Autodesk Inventor part; units mm, degrees
ref_plane "YZ Plane" through (0, 0, 0) normal (1, 0, 0) x (0, 1, 0)
ref_plane "XZ Plane" through (0, 0, 0) normal (0, 1, 0) x (-1, 0, 0)
ref_plane "XY Plane" through (0, 0, 0) normal (0, 0, 1) x (1, 0, 0)
sketch "Boceto1" plane through (0, 0, 0) normal (1, 0, 0) x (0, 1, 0)
  line L0 (-6.321, 6.321) -> (6.321, 6.321) construction
  line L1 (6.321, 6.321) -> (6.321, -6.321) construction
  line L2 (6.321, -6.321) -> (-6.321, -6.321) construction
  line L3 (-6.321, -6.321) -> (-6.321, 6.321) construction
  line L4 (-6.321, 6.321) -> (6.321, -6.321) construction
  line L5 (6.321, 6.321) -> (-6.321, -6.321) construction
  circle A0 centre (6.321, -6.321) radius 0.875
  line L6 (0, 0) -> (7.9878, 0) construction
  circle A1 centre (6.321, 6.321) radius 0.875
  line L7 (0, 0) -> (0, -13.4562) construction
  circle A2 centre (-6.321, -6.321) radius 0.875
  circle A3 centre (-6.321, 6.321) radius 0.875
  circle A4 centre (0, 0) radius 5.5
  line L8 (10, 20) -> (-20, 20)
  line L9 (-20, 20) -> (-20, -20)
  line L10 (-20, -20) -> (10, -20)
  line L11 (10, -20) -> (10, 20)
  dimension "d0" = 12.642
  dimension "d1" = 12.642
  dimension "d2" = 1.75
  dimension "d3" = 11
  dimension "d4" = 30
  dimension "d6" = 20
  dimension "d7" = 10
  dimension "d26" = 20
extrude "Extrusión1" add sketch "Boceto1" along normal blind 2
sketch "Boceto2" plane through (0, -20, -20) normal (0, -1, 0) x (1, 0, 0)
  line L0 (2, 0) -> (2, 40)
  line L1 (2, 40) -> (-38, 40)
  line L2 (-38, 40) -> (-38, 0)
  line L3 (-38, 0) -> (2, 0)
  line L4 (2, 0) -> (2, 40)
  point P0 (0, 20)
  point P1 (2, 0)
  dimension "d10" = 40
  dimension "d11" = 40
extrude "Extrusión2" add sketch "Boceto2" along normal blind 2
fillet "Empalme1" radius 1.5 1 edges at (0, -20, 0)
fillet "Empalme2" radius 1 5 edges at (1, 10, 20) (1, 10, -20) (-38, -21, 20) (-38, -21, -20) (2, -22, 0)
sketch "Boceto4" plane through (0, -20, -20) normal (0, 1, 0) x (1, 0, 0)
  circle A0 centre (-13, -10) radius 2.5
  circle A1 centre (-13, -30) radius 2.5
  circle A2 centre (-28, -10) radius 2.5
  circle A3 centre (-28, -30) radius 2.5
  line L0 (-1.5, -40) -> (-37, -40)
  line L1 (-38, -39) -> (-38, -1)
  point P0 (0, -20)
  dimension "d27" = 5
  dimension "d28" = 5
  dimension "d29" = 5
  dimension "d30" = 5
  dimension "d31" = 10
  dimension "d32" = 20
  dimension "d33" = 20
  dimension "d34" = 15
  dimension "d35" = 10
extrude "Extrusión4" cut sketch "Boceto4" against normal through all
sketch "Boceto3" plane through (0, -20, -20) normal (0, 1, 0) x (1, 0, 0)
  line L0 (0, -40) -> (0, 0)
  line L1 (-28, 0) -> (0, 0)
  line L2 (-28, -40) -> (-28, 0)
  line L3 (0, -40) -> (-28, -40)
  line L4 (-6.125, -3.125) -> (-6.125, -36.875) construction
  line L5 (-7.25, -3.125) -> (-7.25, -36.875)
  line L6 (-5, -36.875) -> (-5, -3.125)
  arc A0 (-5, -3.125) -> (-7.25, -3.125) centre (-6.125, -3.125) ccw
  arc A1 (-7.25, -36.875) -> (-5, -36.875) centre (-6.125, -36.875) ccw
  line L7 (-21.875, -3.125) -> (-21.875, -36.875) construction
  line L8 (-23, -3.125) -> (-23, -36.875)
  line L9 (-20.75, -36.875) -> (-20.75, -3.125)
  arc A2 (-20.75, -3.125) -> (-23, -3.125) centre (-21.875, -3.125) ccw
  arc A3 (-23, -36.875) -> (-20.75, -36.875) centre (-21.875, -36.875) ccw
  point P0 (0, -20)
  point P1 (-6.125, -20)
  point P2 (-21.875, -20)
  point P3 (-21.875, -38)
  point P4 (-21.875, -2)
  point P5 (-6.125, -38)
  point P6 (-6.125, -2)
  dimension "d14" = 2.25
  dimension "d15" = 2.25
  dimension "d16" = 5
  dimension "d17" = 2
  dimension "d18" = 2
  dimension "d19" = 2
  dimension "d20" = 2
  dimension "d21" = 5
properties part number "BRACKET_MOTOR" material "Aluminio 6061"
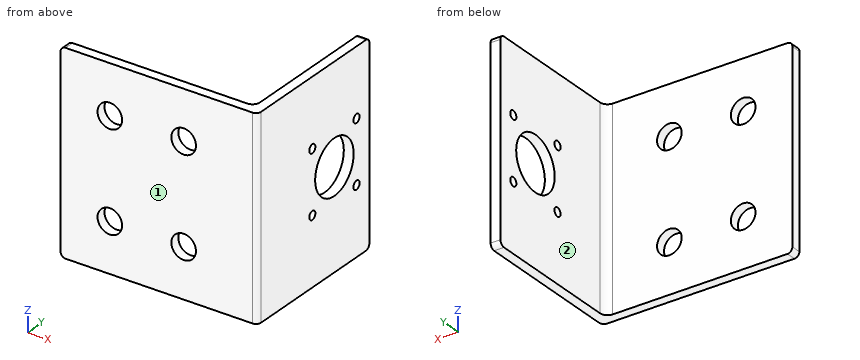
Geometry check sheet. Reference: the model listing, model coordinates, mm. Face numbers are marked on the shaded views. A direction names the side the tool comes from. Give positions to 0.01 mm unless a question says otherwise; leave off trailing zeros. Write each loop counter-clockwise with the first axis right and the second up, starting at its lowest first coordinate (ties: lowest second). Pieces come first, ordered by that corner, then holes. Notation, with made-up numbers: (-27.5, 57) - (-20.5, 57) arc R19 ccw to (-20.5, 62) - close; hole circle Ø11 at (42.25, 47.25). An arc over 180 degrees is marked (long way). Use a Markdown table: item, result.
Q1. Section check D-D, the plane z = 0. Enter the section's corners in (x, y), then the cut area to 3 significant figures.
Computed:
| item | result |
|---|---|
| outline | (-38, -22) - (1, -22) arc R1 ccw to (2, -21) - (2, -5.5) - (0, -5.5) - (0, -18.5) arc R1.5 cw to (-1.5, -20) - (-38, -20) - close; (0, 5.5) - (2, 5.5) - (2, 10) - (0, 10) - close |
| area | 118 mm² |
Q2. Section check C-C, the plane x = -13. Enter the section's corners in (y, z).
Computed:
| item | result |
|---|---|
| outline | (-22, -20) - (-20, -20) - (-20, -12.5) - (-22, -12.5) - close; (-22, -7.5) - (-20, -7.5) - (-20, 7.5) - (-22, 7.5) - close; (-22, 12.5) - (-20, 12.5) - (-20, 20) - (-22, 20) - close |
Q3. Go/stop test with flat-tipped pins: P1, Ø1, axis at x = -32, z = 6.5, coming from the +Y side; P2, Ø14, axis at y = -2.5, z = 2.5, coming from the -X side. Record where each tip stops, or that it passes through.
Computed:
| item | result |
|---|---|
| P1 | stops at y = -20 |
| P2 | stops at x = 0 |
Q4. Section check B-B, the plane y = 0. Enter the section's corners in (x, z), then the cut area to 3 significant figures.
Computed:
| item | result |
|---|---|
| outline | (0, -20) - (2, -20) - (2, -5.5) - (0, -5.5) - close; (0, 5.5) - (2, 5.5) - (2, 20) - (0, 20) - close |
| area | 58.0 mm² |
Q5. Section check A-A, the plane z = 10. Enter the section's corners in (x, y), then the cut area to 3 significant figures.
Computed:
| item | result |
|---|---|
| outline | (-38, -22) - (-30.5, -22) - (-30.5, -20) - (-38, -20) - close; (-25.5, -22) - (-15.5, -22) - (-15.5, -20) - (-25.5, -20) - close; (-10.5, -22) - (1, -22) arc R1 ccw to (2, -21) - (2, 10) - (0, 10) - (0, -18.5) arc R1.5 cw to (-1.5, -20) - (-10.5, -20) - close |
| area | 120 mm² |
Q6. Set-up check for the marked faces 1 and 2: record each of +Z, -Z, +X, -X, +Y, -Y from which the full face is reachable in a straight line by a thin tool's end or side.
Computed:
| item | result |
|---|---|
| face 1 | +Z, -Z, +X, -X, -Y |
| face 2 | +Z, -Z, -X, +Y |
Q7. Thickness scan on L1, parallel to X at y = -20.35, z = -10; L2, parallel to Z at x = -28, y = -21.25; L3, parallel to X at y = -21.5, z = 10. Record the ranges inside material, lowest first. Write a range as [from, to].
Computed:
| item | result |
|---|---|
| L1 | x = [-38, -30.5], [-25.5, -15.5], [-10.5, 2] |
| L2 | z = [-20, -12.5], [-7.5, 7.5], [12.5, 20] |
| L3 | x = [-38, -30.5], [-25.5, -15.5], [-10.5, 1.87] |
